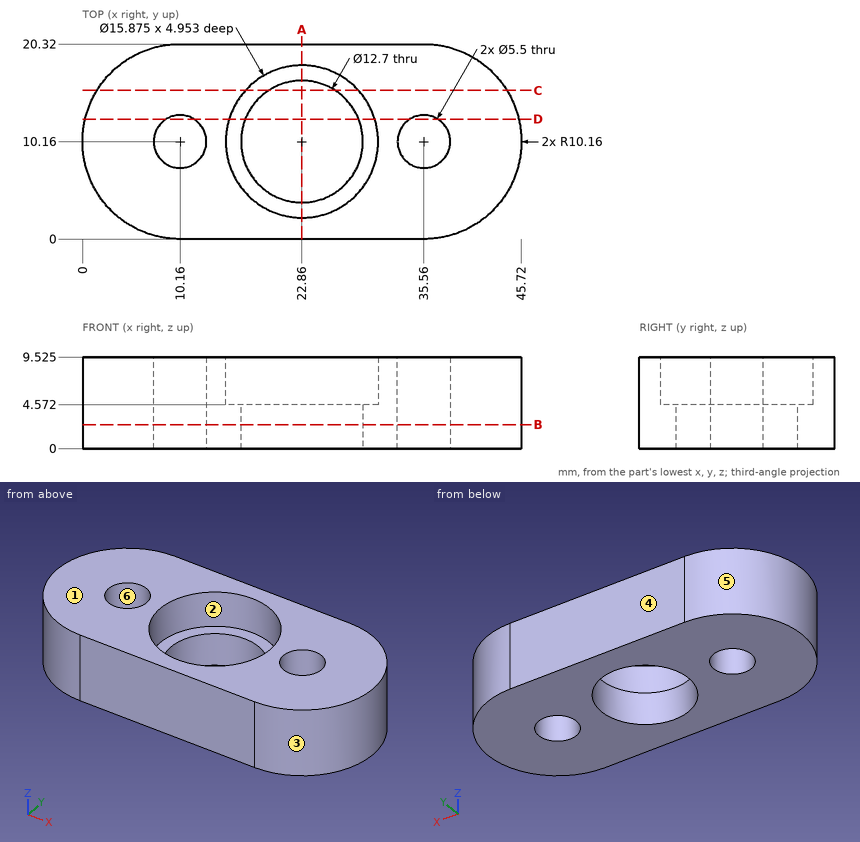
The figure shows three views and two pictorial views of one solid part (mm, origin at its lowest corner). Answer the questions. A direction names the side the tool comes from. Round coordinates to 2 decimals unless told otherwise and drop trailing zeros. Order: outer loops, then holes, each group sorted by start corner. A loop starts at its lowest first (then second) coordinate and runs counter-clockwise, first axis right, second up.
Q1. A cutting plane is placed at B-B, the plane z = 2.5. Determine the outline of the cut face in (x, y).
Solution:
outline: (10.16, 0) - (35.56, 0) arc R10.16 ccw to (35.56, 20.32) - (10.16, 20.32) arc R10.16 ccw to start; hole circle Ø5.5 at (10.16, 10.16); hole circle Ø12.7 at (22.86, 10.16); hole circle Ø5.5 at (35.56, 10.16)
Q2. A cutting plane is placed at D-D, the plane y = 12.5. Determine the outline of the cut face in (x, z) (3 decimals), then the cut area to 3 significant figures.
Solution:
outline: (0.273, 0) - (8.715, 0) - (8.715, 9.525) - (0.273, 9.525) - close; (11.605, 0) - (16.957, 0) - (16.957, 4.572) - (15.275, 4.572) - (15.275, 9.525) - (11.605, 9.525) - close; (28.763, 0) - (34.115, 0) - (34.115, 9.525) - (30.445, 9.525) - (30.445, 4.572) - (28.763, 4.572) - close; (37.005, 0) - (45.447, 0) - (45.447, 9.525) - (37.005, 9.525) - close
area: 246 mm2
Q3. A cutting plane is placed at A-A, the plane x = 22.86. Determine the outline of the cut face in (y, z) (1 decimal).
Solution:
outline: (0, 0) - (3.8, 0) - (3.8, 4.6) - (2.2, 4.6) - (2.2, 9.5) - (0, 9.5) - close; (16.5, 0) - (20.3, 0) - (20.3, 9.5) - (18.1, 9.5) - (18.1, 4.6) - (16.5, 4.6) - close
Q4. A tool of negligible diameter and unlimited length cuts with its end or side. For the marked faces 1 and 2, from which of +Z, -Z, +X, -X, +Y, -Y can it reach the whole face along a straight path? Write none if from no direction.
Solution:
face 1: +Z, +X, -X, +Y, -Y
face 2: +Z
Q5. A cutting plane is placed at C-C, the plane y = 15.5. Determine the outline of the cut face in (x, z) (1 decimal), then the cut area to 3 significant figures.
Solution:
outline: (1.5, 0) - (19.4, 0) - (19.4, 4.6) - (17, 4.6) - (17, 9.5) - (1.5, 9.5) - close; (26.3, 0) - (44.2, 0) - (44.2, 9.5) - (28.7, 9.5) - (28.7, 4.6) - (26.3, 4.6) - close
area: 317 mm2
Q6. Given pin 1 Ø2 at (x, z) = (38, 7) entering from +Y; pin 2 Ø1.5 at (y, z) = (12, 8) entering from +X; pin 3 Ø5 at (y, z) = (15, 2.5) entering from +X, each flat-ended and moving along its own axis, determine where each tip first touches the part or whether it passes through.
Solution:
pin 1: stops at y = 20.22
pin 2: stops at x = 45.66
pin 3: stops at x = 45.45
Q7. The mould has two halves that part along X. Classify the marked faces 3, 4, 5 and 6: pulls with the +X half, pulls with the -X half, needs draft (parallel to the pull), parting line crosses it, or undercut.
Solution:
face 3: pulls with the +X half
face 4: needs draft
face 5: pulls with the -X half
face 6: undercut
Q8. Find the intervals of material crossed by line 1 along X through (y, z) = (11.5, 8); line 2 along Y through (x, z) = (10.16, 2.75); line 3 along X through (y, z) = (12.25, 9.25), in increasing order.
Solution:
line 1: x = 0.09 to 7.76, 12.56 to 15.04, 30.68 to 33.16, 37.96 to 45.63
line 2: y = 0 to 7.41, 12.91 to 20.32
line 3: x = 0.22 to 8.37, 11.95 to 15.2, 30.52 to 33.77, 37.35 to 45.5
